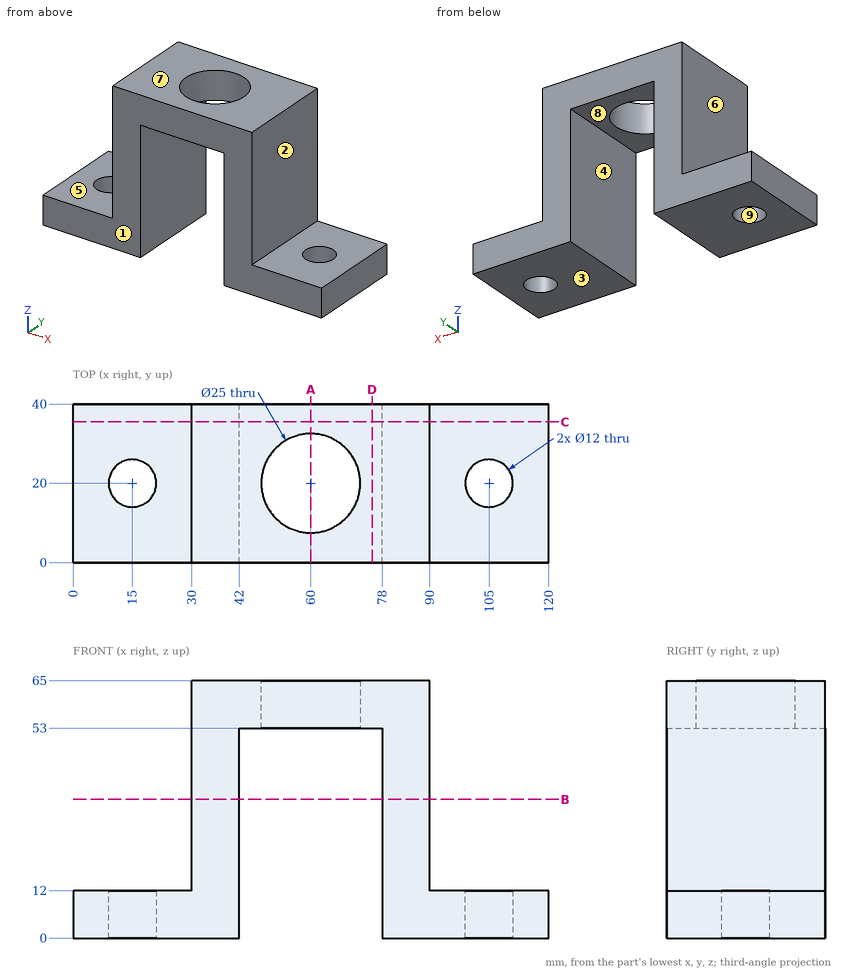
Input: dimensioned drawing with shaded views. Units: mm. Origin: part minimum x, y, z. A direction names the side the tool comes from. Coordinates: 2 decimals unless noted, no trailing zeros. Loops run counter-clockwise (first coordinate to the right, second up) from the corner with the lowest first, then second, coordinate; pieces in that order, holes last. Notation, with made-up numbers: (82.25, 3.25) -> (123.25, 3.25) arc R28 cw to (123.25, 32.25) -> close; hole circle Ø11 at (59, 59.25). An arc over 180 degrees is marked (long way). Use a Markdown table: item, result. Add a question column.
(1) Access query for the marked faces 1, 2, 3, 4 and 5. Directions: +Z, -Z, +X, -X, +Y, -Y. A direction counts if a zero-diameter tool reaches every point of the face in a straight line with its end or side. Return the directions, or none.
(2) Pin query (flat end, axial travel): pin 1 Ø5 at (y, z) = (19, 45.5) entering from +X; pin 2 Ø10 at (y, z) = (16.5, 35.5) entering from -X; pin 3 Ø9 at (x, y) = (109, 11) entering from +Z. Return the tip coordinate at first contact, or that it passes through.
(3) Section query D-D, the plane x = 75.5. Return loops of the section in (y, z), plus the area to 3 significant figures.
(4) Line query: line 1 along X through (y, z) = (21, 25); line 2 along X through (y, z) = (35.5, 5.5); line 3 along Y through (x, z) = (105, 7). Output: solid intervals per line, ascending.
(5) Section query A-A, the plane x = 60. Return loops of the section in (y, z), plus the area to 3 significant figures.
(6) Section query C-C, the plane y = 35.5. Return loops of the section in (x, z), plus the area to 3 significant figures.
(7) Section query B-B, the plane z = 35. Return loops of the section in (x, y).
(8) Mould query, pull axis X, two halves, no side actions, for the marked faces 6, 7, 8 and 9. Classes: pulls with the +X half, pulls with the -X half, needs draft (parallel to the pull), parting line crosses it, or undercut.
Answer:
| question | item | result |
|---|---|---|
| 1 | face 1 | +Z, -Z, +X, -X, -Y |
| 1 | face 2 | +Z, +X, +Y, -Y |
| 1 | face 3 | -Z, +X, -X, +Y, -Y |
| 1 | face 4 | -Z, +Y, -Y |
| 1 | face 5 | +Z, -X, +Y, -Y |
| 2 | pin 1 | stops at x = 90 |
| 2 | pin 2 | stops at x = 30 |
| 2 | pin 3 | stops at z = 12 |
| 3 | outline | (0, 53) -> (40, 53) -> (40, 65) -> (0, 65) -> close |
| 3 | area | 480 mm^2 |
| 4 | line 1 | x = 30 to 42, 78 to 90 |
| 4 | line 2 | x = 0 to 42, 78 to 120 |
| 4 | line 3 | y = 0 to 14, 26 to 40 |
| 5 | outline | (0, 53) -> (7.5, 53) -> (7.5, 65) -> (0, 65) -> close; (32.5, 53) -> (40, 53) -> (40, 65) -> (32.5, 65) -> close |
| 5 | area | 180 mm^2 |
| 6 | outline | (0, 0) -> (42, 0) -> (42, 53) -> (78, 53) -> (78, 0) -> (120, 0) -> (120, 12) -> (90, 12) -> (90, 65) -> (30, 65) -> (30, 12) -> (0, 12) -> close |
| 6 | area | 2,710 mm^2 |
| 7 | outline | (30, 0) -> (42, 0) -> (42, 40) -> (30, 40) -> close; (78, 0) -> (90, 0) -> (90, 40) -> (78, 40) -> close |
| 8 | face 6 | pulls with the -X half |
| 8 | face 7 | needs draft |
| 8 | face 8 | undercut |
| 8 | face 9 | undercut |
